Geometry: final body of the model. Coordinates: model frame, mm. A direction names the side the tool comes from. Give positions to 0.01 mm unless a question says otherwise; leave off trailing zeros. Loops run counter-clockwise (first coordinate to the right, second up) from the corner with the lowest first, then second, coordinate; pieces in that order, holes last.
from build123d import *

# Parameters (mm, degrees)
CROQUIS1_R              = 2.5
SALIENTE_EXTRUIR1_DEPTH = 28
SALIENTE_EXTRUIR3_DEPTH = 2.5
CROQUIS8_R              = 1.5
SALIENTE_EXTRUIR4_DEPTH = 2.5
CROQUIS9_W              = 18
CROQUIS9_H              = 10
SALIENTE_EXTRUIR5_DEPTH = 13
CROQUIS3_W              = 18
CROQUIS3_H              = 14
SALIENTE_EXTRUIR2_DEPTH = 14
CROQUIS4_R              = 5
CORTAR_EXTRUIR1_DEPTH   = 4
CORTAR_EXTRUIR2_START   = -14
CROQUIS4_2_R            = 5
CORTAR_EXTRUIR2_DEPTH   = 4
CORTAR_EXTRUIR3_REACH   = 67.584
CROQUIS5_R              = 3.5
REDONDEO1_R             = 4
CROQUIS10_W             = 40
CROQUIS10_H             = 9
CORTAR_EXTRUIR4_DEPTH   = 20
CROQUIS11_W             = 8
CROQUIS11_H             = 5
SALIENTE_EXTRUIR6_DEPTH = 13
CROQUIS12_R             = 1
CORTAR_EXTRUIR5_DEPTH   = 6
CROQUIS13_W             = 1.6
CROQUIS13_H             = 3.9
CORTAR_EXTRUIR6_DEPTH   = 33
REDONDEO2_R             = 5
REDONDEO3_R             = 12
SALIENTE_EXTRUIR7_START = 3
SALIENTE_EXTRUIR7_DEPTH = 8
CROQUIS16_W             = 2
CROQUIS16_H             = 3
CORTAR_EXTRUIR7_DEPTH   = 2.5


with BuildPart() as part:
    # Croquis1 → Saliente-Extruir1 (new body)
    with BuildSketch(Plane.XY):
        with BuildLine():
            Line((-15.5, 4.5), (15.5, 4.5))
            ThreePointArc((15.5, 4.5), (20, 0), (15.5, -4.5))
            Line((15.5, -4.5), (-15.5, -4.5))
            ThreePointArc((-15.5, -4.5), (-20, 0), (-15.5, 4.5))
        make_face()
        with Locations((-15.5, 0)):
            Circle(CROQUIS1_R, mode=Mode.SUBTRACT)
        with Locations(Location((15.5, 0, 0), (0, 0, 180))):
            Circle(CROQUIS1_R, mode=Mode.SUBTRACT)
    extrude(amount=SALIENTE_EXTRUIR1_DEPTH)

    # Croquis7 → Saliente-Extruir3 (add)
    with BuildSketch(Plane.XY.offset(28)):
        with BuildLine():
            Line((10.434561388, -1.264633608), (10.434561388, -4.5))
            Line((10.434561388, -4.5), (-11.065438612, -4.5))
            Line((-11.065438612, -4.5), (-11.065438612, -1.264634516))
            add(Edge.make_bspline(
                [(-11.065438612, -1.264634516), (-10.873261798, -0.150088047), (-9.571810624, 1.50000001), (-7.999999983, 1.5)],
                knots=[0, 0, 0, 0, 1, 1, 1, 1], degree=3))
            Line((-7.999999983, 1.5), (1e-08, 1.5))
            Line((1e-08, 1.5), (7.369122804, 1.500000949))
            add(Edge.make_bspline(
                [(7.369122804, 1.500000949), (8.940933445, 1.500000937), (10.242384596, -0.150087137), (10.434561388, -1.264633608)],
                knots=[0, 0, 0, 0, 1, 1, 1, 1], degree=3))
        make_face()
    extrude(amount=SALIENTE_EXTRUIR3_DEPTH)

    # Croquis8 → Saliente-Extruir4 (add)
    with BuildSketch(Plane.XY.offset(30.5)):
        with BuildLine():
            Line((15.5, 4.5), (15.5, 39.5))
            Line((15.5, 39.5), (-15.5, 39.5))
            Line((-15.5, 39.5), (-15.5, 4.5))
            ThreePointArc((-15.5, 4.5), (-20, 0), (-15.5, -4.5))
            Line((-15.5, -4.5), (15.5, -4.5))
            ThreePointArc((15.5, -4.5), (20, 0), (15.5, 4.5))
        make_face()
        with Locations((15.5, 0)):
            Circle(CROQUIS8_R, mode=Mode.SUBTRACT)
        with Locations((-15.5, 0)):
            Circle(CROQUIS8_R, mode=Mode.SUBTRACT)
    extrude(amount=SALIENTE_EXTRUIR4_DEPTH)

    # Croquis9 → Saliente-Extruir5 (add)
    with BuildSketch(Plane.XY.offset(33)):
        with Locations((0, 0.5)):
            Rectangle(CROQUIS9_W, CROQUIS9_H)
    extrude(amount=SALIENTE_EXTRUIR5_DEPTH)

    # Croquis3 → Saliente-Extruir2 (add)
    with BuildSketch(Plane.XZ.offset(4.5)):
        with Locations((0, 39)):
            Rectangle(CROQUIS3_W, CROQUIS3_H)
    extrude(amount=SALIENTE_EXTRUIR2_DEPTH)

    # Croquis4 → Cortar-Extruir1 (cut)
    with BuildSketch(Plane.ZY.offset(9)):
        with Locations((39, -11.5)):
            Circle(CROQUIS4_R)
    extrude(amount=-CORTAR_EXTRUIR1_DEPTH, mode=Mode.SUBTRACT)

    # Croquis4<2> → Cortar-Extruir2 (cut)
    with BuildSketch(Plane.ZY.offset(9).offset(CORTAR_EXTRUIR2_START)):
        with Locations((39, -11.5)):
            Circle(CROQUIS4_2_R)
    extrude(amount=-CORTAR_EXTRUIR2_DEPTH, mode=Mode.SUBTRACT)

    # Croquis5 → Cortar-Extruir3 (cut, up to next)
    with BuildSketch(Plane.ZY.offset(5), mode=Mode.PRIVATE) as cortar_extruir3_sk1:
        with Locations((39, -11.5)):
            Circle(CROQUIS5_R)
    cortar_extruir3_tool1 = extrude(cortar_extruir3_sk1.sketch, amount=-CORTAR_EXTRUIR3_REACH, mode=Mode.PRIVATE) & part.part
    add(cortar_extruir3_tool1.solids().sort_by_distance((-5, -11.5, 39))[0], mode=Mode.SUBTRACT)

    # Redondeo1
    redondeo1_edges = [part.edges().sort_by_distance(p)[0] for p in [
        (0, -18.5, 32),
        (0, -18.5, 46),
    ]]
    fillet(redondeo1_edges, radius=REDONDEO1_R)

    # Croquis10 → Cortar-Extruir4 (cut)
    with BuildSketch(Plane(origin=(0, 0, 0), x_dir=(-1, 0, 0), z_dir=(0, 0, -1))):
        Rectangle(CROQUIS10_W, CROQUIS10_H)
    extrude(amount=-CORTAR_EXTRUIR4_DEPTH, mode=Mode.SUBTRACT)

    # Croquis11 → Saliente-Extruir6 (add)
    with BuildSketch(Plane.XY.offset(33)):
        with Locations((-5, 30.65)):
            Rectangle(CROQUIS11_W, CROQUIS11_H)
    extrude(amount=SALIENTE_EXTRUIR6_DEPTH)

    # Croquis12 → Cortar-Extruir5 (cut)
    with BuildSketch(Plane.ZY.offset(9)):
        with Locations(Location((39, 3, 0), (0, 0, 270))):
            Circle(CROQUIS12_R)
        with Locations(Location((39, 30.65, 0), (0, 0, 90))):
            Circle(CROQUIS12_R)
    extrude(amount=-CORTAR_EXTRUIR5_DEPTH, mode=Mode.SUBTRACT)

    # Croquis13 → Cortar-Extruir6 (cut)
    with BuildSketch(Plane(origin=(0, 33.15, 0), x_dir=(1, 0, 0), z_dir=(0, 1, 0))):
        with Locations((-6.614967389, -39)):
            Rectangle(CROQUIS13_W, CROQUIS13_H)
    extrude(amount=-CORTAR_EXTRUIR6_DEPTH, mode=Mode.SUBTRACT)

    # Redondeo2
    redondeo2_edges = [part.edges().sort_by_distance(p)[0] for p in [
        (-15.5, 39.5, 31.75),
        (-15.5, 4.5, 31.75),
        (15.5, 4.5, 31.75),
        (15.5, 39.5, 31.75),
    ]]
    fillet(redondeo2_edges, radius=REDONDEO2_R)

    # Redondeo3
    # the kernel refuses this fillet: 12 mm, written as the material it adds along each edge
    with BuildSketch(Plane(origin=(9, -4.5, 32), x_dir=(0, 0, -1), z_dir=(-1, 0, 0))) as redondeo3_piece_1:
        with BuildLine():
            CenterArc((11.874507866, 12), REDONDEO3_R, 187.180755781, 82.819244219)
            Line((-0.031373033, 10.5), (-1.221961123, 10.35))
            ThreePointArc((-1.221961123, 10.35), (-1.2, 10), (-1.2, 0))
            Line((-1.2, 0), (0, -1.2))
            Line((0, -1.2), (11.874507866, -1.2))
            Line((11.874507866, -1.2), (11.874507866, 0))
        make_face()
    extrude(amount=18)

    # Croquis14 → Saliente-Extruir7 (add)
    with BuildSketch(Plane(origin=(0, 5.5, 0), x_dir=(1, 0, 0), z_dir=(0, 1, 0)).offset(SALIENTE_EXTRUIR7_START)):
        Polygon((10.5, -33), (10.5, -46.00000144), (15.1, -46.00000144), (15.1, -33), (14.1, -33), (14.1, -43.5), (11.5, -43.5), (11.5, -33), align=None)
    extrude(amount=SALIENTE_EXTRUIR7_DEPTH)

    # Croquis16 → Cortar-Extruir7 (cut)
    with BuildSketch(Plane(origin=(0, 0, 30.5), x_dir=(-1, 0, 0), z_dir=(0, 0, -1))):
        with Locations((-5.165983378, 35)):
            Rectangle(CROQUIS16_W, CROQUIS16_H)
        with Locations((5.165983378, 35)):
            Rectangle(CROQUIS16_W, CROQUIS16_H)
    extrude(amount=-CORTAR_EXTRUIR7_DEPTH, mode=Mode.SUBTRACT)


solid = part.part
Item 1: Ray query, probe 1 along Z at (x, y) = (-8.1, 3); probe 2 along X at (y, z) = (0.5, 27.5); probe 3 along Y at (x, z) = (-15.5, 24.5). Return the intervals inside material, ascending.
Values follow:
probe 1: z = 20 to 28, 30.5 to 38, 40 to 46
probe 2: x = -19.97 to -17.95, -13.05 to 13.05, 17.95 to 19.97
probe 3: y = -4.5 to -2.5, 2.5 to 4.5
Item 2: Pin query (flat end, axial travel): pin 1 (9 mm diameter, centred on y = 13.5, z = 39, fed in from -X); pin 2 (1 mm diameter, centred on x = -1.5, y = -9, fed in from -Z); pin 3 (3 mm diameter, centred on y = -2.5, z = 29, fed in from -X). Return the tip coordinate at first contact, or that it passes through.
Values follow:
pin 1: stops at x = 10.5
pin 2: stops at z = 29.07
pin 3: stops at x = -19.78
Item 3: Set-up query: faces 1 (the face through (-7, 31, 40.95)), 2 (the face through (-5, 28.15, 39)), 3 (the face through (4.166, 35, 32)), 4 (the face through (-5, -15, 41)), 5 (the face through (18, 0, 24)). Return all of +Z, -Z, +X, -X, +Y, -Y with unobstructed straight access to the full face (end or side cutting, diameter ignored); none if empty.
Values follow:
face 1: +Y
face 2: +Z, +X, -X
face 3: +Z, -Z
face 4: -X
face 5: -Z
Item 4: Section query B-B on y = 30.65. Return loops of the section in (x, z).
Values follow:
outline: (-15.5, 30.5) - (15.5, 30.5) - (15.5, 33) - (-1, 33) - (-1, 46) - (-9, 46) - (-9, 40) - (-7.41, 40) - (-7.41, 40.95) - (-5.81, 40.95) - (-5.81, 40) - (-3, 40) - (-3, 38) - (-5.81, 38) - (-5.81, 37.05) - (-7.41, 37.05) - (-7.41, 38) - (-9, 38) - (-9, 33) - (-15.5, 33) - close
Item 5: Section query A-A on y = 12.5. Return loops of the section in (x, z).
Values follow:
outline: (-15.5, 30.5) - (15.5, 30.5) - (15.5, 33) - (15.1, 33) - (15.1, 46) - (10.5, 46) - (10.5, 33) - (-15.5, 33) - close; hole (11.5, 33) - (14.1, 33) - (14.1, 43.5) - (11.5, 43.5) - close
Item 6: Draft query along Y for faces 6 (the face through (-5, 33.15, 39)), 7 (the face through (0.13, -17.47, 33.32)), 8 (the face through (13, 12, 46)), 9 (the face through (-3, 31, 39)). Return one class per face: +Y half, -Y half, draft (parallel to the pull), parting line (faces both ways), or undercut.
Values follow:
face 6: +Y half
face 7: -Y half
face 8: draft
face 9: undercut
